Could you check a few things on this model? Use its own coordinates, in mm. Face numbers are marked on the shaded views. A direction names the side the tool comes from. Give positions to 0.01 mm unless a question says otherwise; leave off trailing zeros. Loops run counter-clockwise (first coordinate to the right, second up) from the corner with the lowest first, then second, coordinate; pieces in that order, holes last. Notation, with made-up numbers: (-18.75, 41.25) - (-12.75, 41.25) arc R21 ccw to (-12.75, 78.25) - close; hole circle Ø10 at (41.5, 41.25). An arc over 180 degrees is marked (long way). Write each question's results on one line, items separated by ' | '. Start each with the question number.
(1) I need wall thicknesses on line 1 (Z direction, x = 16, y = 8.5) (1 decimal); line 2 (Y direction, x = 16.25, z = 2.5); line 3 (X direction, y = 38.5, z = 7). Which ranges of each line are inside material? Lowest first, please.
(2) Suppose I cut it at D-D (z = 7.5). Please give me the cut outline in (x, y) (3 decimals), and give its area (3 significant figures).
(3) Suppose I cut it at B-B (z = 3.75). Please give me the cut outline in (x, y), and give its area (3 significant figures).
(4) On a 3-axis mill with a long thin cutter (end or side, diameter ignored), from which of +Z, -Z, +X, -X, +Y, -Y can I reach the whole of each face in a straight line? I mean the marked faces 4 and 5. Say none if no direction works.
(5) If we mould it in two halves opening along X, with no side actions, what happens to the marked faces 1, 2 and 3? For each: released by +X, released by -X, zero draft, split by the parting line, or undercut.
(6) For pin 1 (9.5 mm diameter, centred on x = 11, y = 34, fed in from -Z), with a flat end and sliding along its axis, tell me the tip position at first contact or that it passes through.
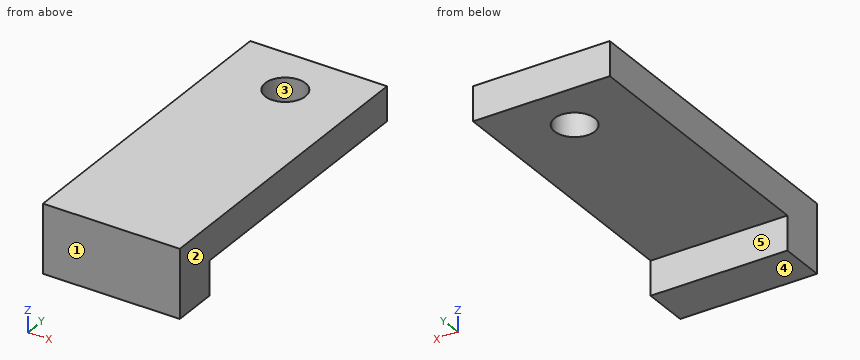
from build123d import *

# Parameters (mm, degrees)
EXTRUDE1_DEPTH         = 19.05
F_10_CLEARANCE_HOLE1_D = 5.6134


with BuildPart() as part:
    # Sketch1 → Extrude1 (new body)
    with BuildSketch(Plane(origin=(0, 0, 0), x_dir=(0, 0, -1), z_dir=(1, 0, 0))):
        Polygon((0, 0), (-9.525, 0), (-9.525, 44.45), (-4.7625, 44.45), (-4.7625, 6.35), (0, 6.35), align=None)
    extrude(amount=EXTRUDE1_DEPTH)

    # #10 Clearance Hole1 (through all)
    with Locations(Plane.XY.offset(9.525)):
        with Locations((9.525, 37.30625)):
            Hole(F_10_CLEARANCE_HOLE1_D / 2)


solid = part.part
Output values:
1) line 1: 4.8 to 9.5 | line 2: 0 to 6.35 | line 3: 0 to 6.98, 12.07 to 19.05
2) outline: (0, 0) - (19.05, 0) - (19.05, 44.45) - (0, 44.45) - close; hole circle Ø5.613 at (9.525, 37.306) | area: 822 mm2
3) outline: (0, 0) - (19.05, 0) - (19.05, 6.35) - (0, 6.35) - close | area: 121 mm2
4) face 4: -Z, +X, -X, +Y, -Y | face 5: -Z, +X, -X, +Y
5) face 1: zero draft | face 2: released by +X | face 3: undercut
6) pin 1: z = 4.76
